For this review, take the finished solid that the model builds, in its own axes (mm). Face numbers are marked on the shaded views. A direction names the side the tool comes from. Give positions to 0.01 mm unless a question says otherwise; leave off trailing zeros. Write each loop counter-clockwise with the first axis right and the second up, starting at its lowest first coordinate (ties: lowest second). Pieces come first, ordered by that corner, then holes.
1) We need section C-C on x = 0. Give the number of separate pieces and of enclosed holes in the cut face, and give its area (3 significant figures).
2) Wall thickness on line 1 along Y through (x, z) = (9, -4.75); line 2 along Y through (x, z) = (0, -3.85); line 3 along X through (y, z) = (-3.75, 0): over which ranges is each line inside the solid? List them lowest first.
3) We need section B-B on y = -8. Give the boundary of the cut face in (x, z).
4) Draft analysis for pull direction X (two halves, no side actions). For the marked faces 3, 4 and 5, state which applies: pulls with the +X half, pulls with the -X half, needs draft (parallel to the pull), parting line crosses it, or undercut.
5) For P1, Ø1.5, axis at y = -6, z = -1.5, coming from the +X side; P2, Ø1, axis at y = -3.5, z = -4, coming from the -X side; P3, Ø6, axis at y = -10, z = -5, coming from the +X side; P4, Ø4, axis at x = -8.5, y = -7, coming from the -Z side, all flat-tipped, find the tip position at first contact; note any pin that passes through.
6) Machinability: for the marked faces 1 and 2, which of the approach directions +Z, -Z, +X, -X, +Y, -Y give a long, thin tool a straight path to every point of the face, cutting with its end or side? Answer none if there is none.
7) We need section D-D on y = 2.5. Give the boundary of the cut face in (x, z).
from build123d import *

# Parameters (mm, degrees)
SKETCH_1_R               = 10
EXTRUDE_1_DEPTH          = 4
SKETCH_2_R               = 12
EXTRUDE_2_DEPTH          = 2
EXTRUDE_START            = 2
SKETCH_3_R               = 12
EXTRUDE_3_DEPTH          = 2
SKETCH_4_R               = 5
EXTRUDE_4_DEPTH          = 10
SKETCH_5_R               = 2
CUT_EXTRUDE_1_DEPTH      = 25.738633754
FILLET_2_R               = 1
CUT_EXTRUDE_2_DEPTH      = 10
CUT_EXTRUDE_2_DEPTH_BACK = 10
SKETCH_6_R               = 1.5


with BuildPart() as part:
    # 草图1 → 凸台-拉伸1 (new body)
    with BuildSketch(Plane(origin=(0, 0, 0), x_dir=(1, 0, 0), z_dir=(0, 1, 0))):
        with Locations(Location((0, 0, 0), (0, 0, 270))):
            Circle(SKETCH_1_R)
    extrude(amount=EXTRUDE_1_DEPTH)

    # 草图2 → 凸台-拉伸2 (add)
    with BuildSketch(Plane(origin=(0, 4, 0), x_dir=(1, 0, 0), z_dir=(0, 1, 0))):
        with Locations(Location((0, 0, 0), (0, 0, 270))):
            Circle(SKETCH_2_R)
    extrude(amount=EXTRUDE_2_DEPTH)

    # 草图3 → 凸台-拉伸3 (add)
    with BuildSketch(Plane.XZ.offset(EXTRUDE_START)):
        with Locations(Location((0, 0, 0), (0, 0, 90))):
            Circle(SKETCH_3_R)
    extrude(amount=-EXTRUDE_3_DEPTH)

    # 草图4 → 凸台-拉伸4 (add)
    with BuildSketch(Plane(origin=(0, -2, 0), x_dir=(-1, 0, 0), z_dir=(0, -1, 0))):
        with Locations(Location((0, 0, 0), (0, 0, 90))):
            Circle(SKETCH_4_R)
    extrude(amount=EXTRUDE_4_DEPTH)

    # 草图5 → 切除-拉伸1 (cut, through all)
    with BuildSketch(Plane.XZ.offset(12)):
        with Locations(Location((0, 0, 0), (0, 0, 270))):
            Circle(SKETCH_5_R)
    extrude(amount=-CUT_EXTRUDE_1_DEPTH, mode=Mode.SUBTRACT)

    # 圆角2
    fillet_2_edges = [part.edges().sort_by_distance(p)[0] for p in [
        (0, -2, -12),
        (0, 4, -12),
        (0, 6, -12),
        (0, 0, -12),
    ]]
    fillet(fillet_2_edges, radius=FILLET_2_R - 0.0001)  # a hair under: the kernel refuses the full size

    # 草图6 → 切除-拉伸2 (cut, two sides: drawn at the far end of the back side and taken through both)
    with BuildSketch(Plane.XY.offset(-CUT_EXTRUDE_2_DEPTH_BACK)):
        with Locations((0, -8)):
            Circle(SKETCH_6_R)
    extrude(amount=CUT_EXTRUDE_2_DEPTH + CUT_EXTRUDE_2_DEPTH_BACK, mode=Mode.SUBTRACT)


solid = part.part
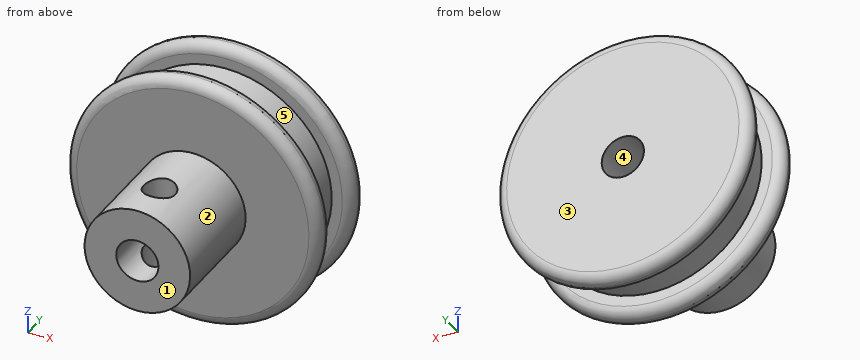
Results list:
1. separate pieces: 4
1. enclosed holes: 0
1. area: 184 mm2
2. line 1: y = -2 to 0, 4 to 6
2. line 2: y = -12 to -9.5, -6.5 to 6
2. line 3: x = -5 to -2, 2 to 5
3. outline: (-1.5, -4.77) - (-1.5, -1.32) arc R2 cw to (-1.5, 1.32) - (-1.5, 4.77) arc R5 ccw to start; (1.5, -4.77) arc R5 ccw to (1.5, 4.77) - (1.5, 1.32) arc R2 cw to (1.5, -1.32) - close
4. face 3: needs draft
4. face 4: undercut
4. face 5: parting line crosses it
5. P1: stops at x = 4.94
5. P2: stops at x = -3.57
5. P3: stops at x = 4.58
5. P4: passes through
6. face 1: +Z, -Z, +X, -X, -Y
6. face 2: -Y
7. outline: circle Ø20 at (0, 0); hole circle Ø4 at (0, 0)
